```python
from build123d import *

# Parameters (mm, degrees)
SKETCH012_R             = 105
SKETCH012_R_2           = 85
PAD006_DEPTH            = 20
PAD005_DEPTH            = 20
POCKET006_DEPTH         = 10
SKETCH013_R             = 1.6
POCKET007_DEPTH         = 20
POCKET008_DEPTH         = 3
FILLET001_R             = 9
BODY002_PLACEMENT_ANGLE = 30


with BuildPart() as part:
    # Sketch012 → Pad006 (new body)
    with BuildSketch(Plane.XY):
        Circle(SKETCH012_R)
        Circle(SKETCH012_R_2, mode=Mode.SUBTRACT)
    extrude(amount=PAD006_DEPTH)

    # Sketch014 → Pad005 (join)
    with BuildSketch(Plane.XY):
        with BuildLine():
            ThreePointArc((-28.284271, -10), (-21.213203, -21.213203), (-10, -28.284271))
            Line((-10, -100), (-10, -28.284271))
            Line((10, -100), (-10, -100))
            Line((10, -28.284271), (10, -100))
            ThreePointArc((10, -28.284271), (21.213203, -21.213203), (28.284271, -10))
            Line((100, -10), (28.284271, -10))
            Line((100, 10), (100, -10))
            Line((28.284271, 10), (100, 10))
            ThreePointArc((28.284271, 10), (0, 30), (-28.284271, 10))
            Line((-100, 10), (-28.284271, 10))
            Line((-100, -10), (-100, 10))
            Line((-28.284271, -10), (-100, -10))
        make_face()
    extrude(amount=PAD005_DEPTH)

    # Sketch011 → Pocket006 (cut)
    with BuildSketch(Plane.XY):
        Polygon((19.052559, 11), (0, 22), (-19.052559, 11), (-19.052559, -11), (0, -22), (19.052559, -11), align=None)
    extrude(amount=POCKET006_DEPTH, mode=Mode.SUBTRACT)

    # Sketch013 → Pocket007 (cut)
    with BuildSketch(Plane.XY):
        with Locations((-13, 0)):
            Circle(SKETCH013_R)
        with Locations((13, 0)):
            Circle(SKETCH013_R)
    extrude(amount=POCKET007_DEPTH, mode=Mode.SUBTRACT)

    # Sketch015 → Pocket008 (cut)
    with BuildSketch(Plane.XY.offset(20)):
        Polygon((21.650635, 12.5), (0, 25), (-21.650635, 12.5), (-21.650635, -12.5), (0, -25), (21.650635, -12.5), align=None)
    extrude(amount=-POCKET008_DEPTH, mode=Mode.SUBTRACT)

    # Fillet001
    fillet001_edges = [part.edges().sort_by_distance(p)[0] for p in [
        (-105, 0, 20),
        (-105, 0, 0),
    ]]
    fillet(fillet001_edges, radius=FILLET001_R)


with BuildPart() as part_1:
    # Body002 placement: moved
    add(part.part.moved(Location((50, 50, 100))).rotate(Axis((50, 50, 100), (0, 0, 1)), BODY002_PLACEMENT_ANGLE))


solid = part_1.part
```
The model under review builds one solid part; all positions refer to its coordinate system, in mm. A direction names the side the tool comes from. Round coordinates to 2 decimals unless told otherwise and drop trailing zeros. Loops run counter-clockwise (first coordinate to the right, second up) from the corner with the lowest first, then second, coordinate; pieces in that order, holes last. Notation, with made-up numbers: (-33.5, -21) -> (-18.5, -21) arc R27 cw to (-18.5, 9) -> close; hole circle Ø4 at (8.25, -25). An arc over 180 degrees is marked (long way). Answer as a JSON object with one key per item and string values. Group by question number.
1) Mouldability with a two-part tool opening along Y and no side actions: class faces 4 (the face through (81.54, -50.15, 109.99)), 5 (the face through (131.895, 27.234, 109.86)) as released by +Y, released by -Y, zero draft, split by the parting line, or undercut.
2) We need section A-A on x = 50. Write out the cut boundary in (y, z), then the cut area to 3 significant figures.
3) For line 1 (X direction, y = 56.5, z = 113.5); line 2 (X direction, y = 77, z = 115.5); line 3 (Y direction, x = 24, z = 112.25), list the stretches that pass through material, from the lowest coordinate up. Write a range as [from, to].
4) We need section B-B on z = 102.75. Write out the cut boundary in (x, y).
5) For faces 1 (the face through (66.4, 40.3, 104.9)), 2 (the face through (68.66, 39.02, 118.52)), 3 (the face through (-4.14, 30.29, 109.86)), list the 3-axis set-ups (+Z, -Z, +X, -X, +Y, -Y) from which the entire face can be reached by the end or side of a thin tool; tool diameter is ignored.
6) We need section C-C on y = 35. Give the number of separate pieces and of enclosed holes in the cut face, then the cut area to 3 significant figures.
7) For pin 1 Ø12 at (x, z) = (22.5, 103) entering from +Y; pin 2 Ø0.9 at (x, z) = (47, 119) entering from -Y; pin 3 Ø13 at (x, y) = (37.5, 58) entering from +Z, all flat-tipped, find the tip position at first contact; note any pin that passes through.
Result set:
{
 "1": {"face 4": "split by the parting line", "face 5": "undercut"},
 "2": {"outline": "(-55, 109) arc R9 ccw to (-46, 100) -> (-35, 100) -> (-35, 120) -> (-46, 120) arc R9 ccw to (-55, 111) -> close; (20, 100) -> (30.95, 100) -> (30.95, 110) -> (69.05, 110) -> (69.05, 100) -> (80, 100) -> (80, 120) -> (71.65, 120) -> (71.65, 117) -> (28.35, 117) -> (28.35, 120) -> (20, 120) -> close; (135, 100) -> (146, 100) arc R9 ccw to (155, 109) -> (155, 111) arc R9 ccw to (146, 120) -> (135, 120) -> close", "area": "1,420 mm²"},
 "3": {"line 1": "[-54.44, -34.75], [20.71, 59.66], [62.86, 81.26], [134.75, 154.44]", "line 2": "[-50.22, -30.6], [36.92, 63.08], [76.77, 116.77], [130.6, 150.22]", "line 3": "[-51.64, -30.93], [23.44, 64.97], [130.93, 151.64]"},
 "4": {"outline": "circle Ø204.95 at (50, 50); hole (-28.1, 16.46) -> (20.51, 44.52) arc R30 cw to (69.49, 72.8) -> (118.1, 100.87) arc R85 ccw to start; hole (-18.1, -0.87) arc R85 ccw to (83.54, -28.1) -> (55.48, 20.51) arc R30 cw to (30.51, 27.2) -> close; hole (28, 50) -> (39, 30.95) -> (61, 30.95) -> (72, 50) -> (61, 69.05) -> (39, 69.05) -> close; hole (72.8, 30.51) -> (100.87, -18.1) arc R85 ccw to (128.1, 83.54) -> (79.49, 55.48) arc R30 cw to start"},
 "5": {"face 1": "-Z", "face 2": "+Z", "face 3": "+Z, -Z"},
 "6": {"separate pieces": "3", "enclosed holes": "0", "area": "1,810 mm²"},
 "7": {"pin 1": "y = 152.22", "pin 2": "y = -50.85", "pin 3": "z = 117"}
}
